```python
from build123d import *

# Parameters (mm, degrees)
F0_W      = 60.96
F0_H      = 57.785
F1_DEPTH  = 15.875
F2_W      = 57.15
F2_H      = 53.975
F3_DEPTH  = 12.7
F4_R      = 3.4925
F4_R_2    = 5.3975
F5_DEPTH  = 15.876
F6_W      = 12.7
F6_H      = 8.255
F7_DEPTH  = 3.175
F4_W      = 11.43
F4_H      = 12.7
F10_DEPTH = 25.4
F11_R     = 1.5875
F12_W     = 20.32
F12_H     = 25.4
F12_R     = 2.5527
F13_DEPTH = 15.875
F14_R     = 3.175
F15_R     = 1.58749
F16_W     = 3.175
F16_H     = 12.7
F17_DEPTH = 1.905


# Not quite as in the source:
# - a fillet or chamfer is up to 0.001 mm smaller than in the source, because OpenCascade refuses the exact size
# - a feature names something its author has since deleted; it is built from what else it names


with BuildPart() as f1:
    # F0 (on Top) → F1 (new body)
    with BuildSketch(Plane.XY):
        with Locations((30.48, 28.8925)):
            Rectangle(F0_W, F0_H)
    extrude(amount=F1_DEPTH)

    # F2 (on face) → F3 (cut)
    with BuildSketch(Plane.XY.offset(15.875)):
        with Locations((30.48, 28.8925)):
            Rectangle(F2_W, F2_H)
    extrude(amount=-F3_DEPTH, mode=Mode.SUBTRACT)

    # F4 (on face) → F5 (cut, through all)
    with BuildSketch(Plane(origin=(0, 0, 0), x_dir=(1, 0, 0), z_dir=(0, 0, -1))):
        with Locations((17.145, -45.085)):
            Circle(F4_R)
        with Locations((50.165, -45.085)):
            Circle(F4_R_2)
        with BuildLine():
            Line((37.1475, -5.08), (23.8125, -5.08))
            ThreePointArc((23.8125, -5.08), (22.6899679849, -5.5449679849), (22.225, -6.6675))
            Line((22.225, -6.6675), (22.225, -30.1625))
            ThreePointArc((22.225, -30.1625), (22.6899679849, -31.2850320151), (23.8125, -31.75))
            Line((23.8125, -31.75), (37.1475, -31.75))
            ThreePointArc((37.1475, -31.75), (38.2700320151, -31.2850320151), (38.735, -30.1625))
            Line((38.735, -30.1625), (38.735, -6.6675))
            ThreePointArc((38.735, -6.6675), (38.2700320151, -5.5449679849), (37.1475, -5.08))
        make_face()
    extrude(amount=-F5_DEPTH, mode=Mode.SUBTRACT)

    # F6 (on face) → F7 (join)
    with BuildSketch(Plane.XY.offset(3.175)):
        with Locations((8.255, 16.8275)):
            Rectangle(F6_W, F6_H)
        with Locations((52.705, 16.8275)):
            Rectangle(F6_W, F6_H)
    extrude(amount=F7_DEPTH)

    # F4 (on face) → F10 (cut)
    with BuildSketch(Plane(origin=(0, 0, 0), x_dir=(1, 0, 0), z_dir=(0, 0, -1))):
        with Locations((36.195, -51.435)):
            Rectangle(F4_W, F4_H)
    extrude(amount=-F10_DEPTH, mode=Mode.SUBTRACT)

    # F11
    f11_edges = [f1.edges().sort_by_distance(p)[0] for p in [
        (0, 57.785, 7.9375),
        (0, 0, 7.9375),
        (60.96, 57.785, 7.9375),
        (60.96, 0, 7.9375),
    ]]
    fillet(f11_edges, radius=F11_R)

    # F12 (on Top) → F13 (join, through all)
    with BuildSketch(Plane.XY):
        with Locations((-10.16, 26.9875)):
            Rectangle(F12_W, F12_H)
        with Locations((-9.525, 26.9875)):
            Circle(F12_R, mode=Mode.SUBTRACT)
        Polygon((-12.1739487758, 20.6375), (-1.27, 20.6375), (-1.27, 17.4625), (-15.3489487758, 17.4625), (-17.145, 17.4625), (-17.145, 19.2585512242), (-17.145, 34.7164487758), (-17.145, 36.5125), (-15.3489487758, 36.5125), (-1.27, 36.5125), (-1.27, 33.3375), (-12.1739487758, 33.3375), (-13.97, 33.3375), (-13.97, 31.5414487758), (-13.97, 22.4335512242), (-13.97, 20.6375), align=None, mode=Mode.SUBTRACT)
        with Locations((71.12, 26.9875)):
            Rectangle(F12_W, F12_H)
        with Locations((68.58, 26.9875)):
            Circle(F12_R, mode=Mode.SUBTRACT)
        Polygon((76.3089487758, 17.4625), (62.23, 17.4625), (62.23, 20.6375), (73.1339487758, 20.6375), (74.93, 20.6375), (74.93, 22.4335512242), (74.93, 31.5414487758), (74.93, 33.3375), (73.1339487758, 33.3375), (62.23, 33.3375), (62.23, 36.5125), (76.3089487758, 36.5125), (78.105, 36.5125), (78.105, 34.7164487758), (78.105, 19.2585512242), (78.105, 17.4625), align=None, mode=Mode.SUBTRACT)
        Polygon((73.1339487758, 20.6375), (76.3089487758, 17.4625), (78.105, 17.4625), (78.105, 19.2585512242), (74.93, 22.4335512242), (74.93, 20.6375), align=None)
        Polygon((74.93, 31.5414487758), (78.105, 34.7164487758), (78.105, 36.5125), (76.3089487758, 36.5125), (73.1339487758, 33.3375), (74.93, 33.3375), align=None)
        Polygon((-17.145, 34.7164487758), (-13.97, 31.5414487758), (-13.97, 33.3375), (-12.1739487758, 33.3375), (-15.3489487758, 36.5125), (-17.145, 36.5125), align=None)
        Polygon((-15.3489487758, 17.4625), (-12.1739487758, 20.6375), (-13.97, 20.6375), (-13.97, 22.4335512242), (-17.145, 19.2585512242), (-17.145, 17.4625), align=None)
    extrude(amount=F13_DEPTH)

    # F14
    f14_edges = [f1.edges().sort_by_distance(p)[0] for p in [
        (-20.32, 14.2875, 7.9375),
        (0, 14.2875, 7.9375),
        (-20.32, 39.6875, 7.9375),
        (0, 39.6875, 7.9375),
        (60.96, 14.2875, 7.9375),
        (81.28, 14.2875, 7.9375),
        (81.28, 39.6875, 7.9375),
        (60.96, 39.6875, 7.9375),
    ]]
    fillet(f14_edges, radius=F14_R)

    # F15 (radius 1.5875 in the source; OpenCascade refuses exactly that, so slightly less here)
    f15_edges = [f1.edges().sort_by_distance(p)[0] for p in [
        (62.23, 17.4625, 7.9375),
        (62.23, 20.6375, 7.9375),
        (62.23, 33.3375, 7.9375),
        (62.23, 36.5125, 7.9375),
        (76.308949, 17.4625, 7.9375),
        (78.105, 19.258551, 7.9375),
        (78.105, 34.716449, 7.9375),
        (74.93, 31.541449, 7.9375),
        (74.93, 22.433551, 7.9375),
        (73.133949, 20.6375, 7.9375),
        (73.133949, 33.3375, 7.9375),
        (76.308949, 36.5125, 7.9375),
        (-1.27, 33.3375, 7.9375),
        (-1.27, 36.5125, 7.9375),
        (-15.348949, 36.5125, 7.9375),
        (-12.173949, 33.3375, 7.9375),
        (-15.348949, 17.4625, 7.9375),
        (-12.173949, 20.6375, 7.9375),
        (-1.27, 17.4625, 7.9375),
        (-1.27, 20.6375, 7.9375),
        (-17.145, 19.258551, 7.9375),
        (-13.97, 22.433551, 7.9375),
        (-17.145, 34.716449, 7.9375),
        (-13.97, 31.541449, 7.9375),
    ]]
    fillet(f15_edges, radius=F15_R)

    # F16 (on face) → F17 (cut, through all)
    with BuildSketch(Plane.XZ):
        with Locations((15.875, 9.525)):
            Rectangle(F16_W, F16_H)
        with Locations((45.085, 9.525)):
            Rectangle(F16_W, F16_H)
    extrude(amount=-F17_DEPTH, mode=Mode.SUBTRACT)


solid = f1.part
```
Part model, mm, in its own coordinate system. A direction names the side the tool comes from. Round coordinates to 2 decimals unless told otherwise and drop trailing zeros. Write each loop counter-clockwise with the first axis right and the second up, starting at its lowest first coordinate (ties: lowest second). Pieces come first, ordered by that corner, then holes. Notation, with made-up numbers: (-38, -1.75) -> (-13, -1.75) arc R8 ccw to (-13, 12.25) -> close; hole circle Ø7 at (-24.5, 50.5). An arc over 180 degrees is marked (long way). Return JSON: item names as keys, results as strings. Group by question number.
Q1. Pin check, flat tips, straight feed: pin 1 (2.5 mm diameter, centred on x = -5.5, z = 7.5, fed in from -Y); pin 2 (4 mm diameter, centred on y = 48, z = 7, fed in from +X); pin 3 (9.5 mm diameter, centred on x = 67, z = 10, fed in from -Y). Stop position of each tip, or through.
Q2. Saw through at D-D on z = 12.75. State how many separate pieces and enclosed holes the cut face has, plus the area to 3 significant figures.
Q3. Mould opens along X. For faces 1 (the flat face through (60.96, 6, 8)), 2 (the flat face through (30, 1, 15.875)), 3 (the cylindrical face through (-0.91, 40.64, 8.05)), 4 (the cylindrical face through (-8.35, 24.72, 7.83)) say: pulls with the +X half, pulls with the -X half, needs draft (parallel to the pull), parting line crosses it, or undercut.
Q4. Saw through at C-C on y = 46.5. Write the cut outline in (x, z) (3 decimals), plus the area to 3 significant figures.
Q5. Which spindle directions (+Z, -Z, +X, -X, +Y, -Y) get a long thin tool onto all of the face, cutting with end or side? Do faces 5 (the flat face through (36, 45.085, 2)), 6 (the flat face through (8, 1.905, 10)), 7 (the flat face through (-7, 17.462, 8)). Say none if no direction does.
Q6. Probe L1, parallel to Y at x = 68.58, z = 12; L2, parallel to Y at x = 2.5, z = 6 (3 decimals); L3, parallel to X at y = 48.5, z = 7 (3 decimals). List the from-to ranges inside material, lowest first. Write a range as [from, to].
Q7. Saw through at B-B on y = 16. Write the cut outline in (x, z) (3 decimals).
Q8. Saw through at A-A on x = 68.58. Write the cut outline in (y, z) (1 decimal), plus the area to 3 significant figures.
Answer:
{
 "1": {"pin 1": "y = 14.29", "pin 2": "x = 60.96", "pin 3": "y = 13.67"},
 "2": {"separate pieces": "3", "enclosed holes": "8", "area": "1,190 mm2"},
 "3": {"face 1": "pulls with the +X half", "face 2": "needs draft", "face 3": "pulls with the -X half", "face 4": "undercut"},
 "4": {"outline": "(0, 0) -> (13.952, 0) -> (13.952, 3.175) -> (1.905, 3.175) -> (1.905, 15.875) -> (0, 15.875) -> close; (20.338, 0) -> (30.48, 0) -> (30.48, 3.175) -> (20.338, 3.175) -> close; (41.91, 0) -> (44.956, 0) -> (44.956, 3.175) -> (41.91, 3.175) -> close; (55.374, 0) -> (60.96, 0) -> (60.96, 15.875) -> (59.055, 15.875) -> (59.055, 3.175) -> (55.374, 3.175) -> close", "area": "152 mm2"},
 "5": {"face 5": "+Z, -Z, +Y", "face 6": "+Z", "face 7": "+Z, -Z"},
 "6": {"L1": "[14.29, 17.46], [20.64, 24.43], [29.54, 33.34], [36.51, 39.69]", "L2": "[0, 1.905], [12.7, 20.955], [55.88, 57.785]", "L3": "[0, 1.905], [59.055, 60.96]"},
 "7": {"outline": "(-19.963, 0) -> (22.225, 0) -> (22.225, 3.175) -> (14.605, 3.175) -> (14.605, 6.35) -> (1.905, 6.35) -> (1.905, 15.875) -> (-19.963, 15.875) -> close; (38.735, 0) -> (80.923, 0) -> (80.923, 15.875) -> (59.055, 15.875) -> (59.055, 6.35) -> (46.355, 6.35) -> (46.355, 3.175) -> (38.735, 3.175) -> close"},
 "8": {"outline": "(14.3, 0) -> (17.5, 0) -> (17.5, 15.9) -> (14.3, 15.9) -> close; (20.6, 0) -> (24.4, 0) -> (24.4, 15.9) -> (20.6, 15.9) -> close; (29.5, 0) -> (33.3, 0) -> (33.3, 15.9) -> (29.5, 15.9) -> close; (36.5, 0) -> (39.7, 0) -> (39.7, 15.9) -> (36.5, 15.9) -> close", "area": "221 mm2"}
}
